The listing builds one solid part. Answer for the finished solid, in the listing's coordinates (mm). Round coordinates to 2 decimals unless told otherwise and drop trailing zeros. Write each loop counter-clockwise with the first axis right and the second up, starting at its lowest first coordinate (ties: lowest second). Pieces come first, ordered by that corner, then holes. Notation, with made-up numbers: M 32.25,13 L 40.25,13 A34 ccw 40.25,48 Z; hole C 71,19.5 d9. An arc over 180 degrees is marked long. Answer as CSV lines item,"result". Start each with the question number.
from build123d import *

# Parameters (mm, degrees)
F0_R     = 75
F1_DEPTH = 15
F2_R     = 6.2
F3_DEPTH = 25
F4_R     = 25
F5_DEPTH = 25


with BuildPart() as f1:
    # F0 (on Top) → F1 (new body)
    with BuildSketch(Plane.XY):
        Circle(F0_R)
    extrude(amount=F1_DEPTH)

    # F2 (on face) → F3 (cut)
    with BuildSketch(Plane.XY.offset(15)):
        with Locations((0, 51.259788)):
            Circle(F2_R)
        with Locations((-35.355339, -34.095551)):
            Circle(F2_R)
        with Locations((-50, 1.259788)):
            Circle(F2_R)
        with Locations((-35.355339, 36.615127)):
            Circle(F2_R)
        with Locations((0, -48.740212)):
            Circle(F2_R)
        with Locations((35.355339, -34.095551)):
            Circle(F2_R)
        with Locations((50, 1.259788)):
            Circle(F2_R)
        with Locations((35.355339, 36.615127)):
            Circle(F2_R)
    extrude(amount=-F3_DEPTH, mode=Mode.SUBTRACT)

    # F4 (on face) → F5 (cut)
    with BuildSketch(Plane.XY.offset(15)):
        Circle(F4_R)
    extrude(amount=-F5_DEPTH, mode=Mode.SUBTRACT)


solid = f1.part
Q1. Each of these flat-tipped pins is pushed along its axis until it touches: P1, Ø6, axis at y = 43, z = 12.5, coming from the +X side; P2, Ø8, axis at x = 1.5, z = 8.5, coming from the -Y side; P3, Ø3, axis at x = 56.5, z = 4.5, coming from the -Y side. Where does it stop, or does it pass through?
Q2. Find section A-A (x = 0). Determine the outline of the cut face in (y, z), plus the area to 3 significant figures.
Q3. Find section B-B (y = 9.5). Determine the outline of the cut face in (x, z), plus the area to 3 significant figures.
Q4. Find section D-D (z = 12). Count the separate pieces of the cut face and the enclosed holes in it, plus the area to 3 significant figures.
Q5. Find section C-C (x = -50). Determine the outline of the cut face in (y, z).
Q6. Straight lines are drawn through the part: L1, parallel to X at y = 41.5, z = 11.25; L2, parallel to X at y = 33, z = 12.25; L3, parallel to X at y = 3, z = 10. For each, find the intervals that lie inside material, in ascending order.
Q7. The mould has two halves that part along X. Classify faces 1 (the face through (-1.344, -54.793, 7.605)), 2 (the face through (-9.764, 74.362, 7.395)), 3 (the face through (-18, 18, 15)): +X half, -X half, draft (parallel to the pull), parting line (faces both ways), or undercut.
Reported:
1,P1,"stops at x = 63.44"
1,P2,"stops at y = -75"
1,P3,"stops at y = -50.99"
2,outline,"M -75,0 L -54.94,0 L -54.94,15 L -75,15 Z; M -42.54,0 L -25,0 L -25,15 L -42.54,15 Z; M 25,0 L 45.06,0 L 45.06,15 L 25,15 Z; M 57.46,0 L 75,0 L 75,15 L 57.46,15 Z"
2,area,"1,130 mm2"
3,outline,"M -74.4,0 L -23.12,0 L -23.12,15 L -74.4,15 Z; M 23.12,0 L 74.4,0 L 74.4,15 L 23.12,15 Z"
3,area,"1,540 mm2"
4,separate pieces,"1"
4,enclosed holes,"9"
4,area,"14,700 mm2"
5,outline,"M -55.9,0 L -4.94,0 L -4.94,15 L -55.9,15 Z; M 7.46,0 L 55.9,0 L 55.9,15 L 7.46,15 Z"
6,L1,"x = -62.47 to -39.17, -31.54 to 31.54, 39.17 to 62.47"
6,L2,"x = -67.35 to -40.39, -30.32 to 30.32, 40.39 to 67.35"
6,L3,"x = -74.94 to -55.95, -44.05 to -24.82, 24.82 to 44.05, 55.95 to 74.94"
7,face 1,"undercut"
7,face 2,"parting line"
7,face 3,"draft"
